CAD build for the part. Positions are in the model's coordinates, mm. A direction names the side the tool comes from. Give positions to 0.01 mm unless a question says otherwise; leave off trailing zeros. Write each loop counter-clockwise with the first axis right and the second up, starting at its lowest first coordinate (ties: lowest second). Pieces come first, ordered by that corner, then holes. Notation, with made-up numbers: M 23,43.5 L 35,43.5 A24 cw 35,76.5 Z; hole C 33,85 d7. An arc over 180 degrees is marked long. One line per question, with ' | ' between items. Start each with the question number.
1. Wall check: L1, parallel to Y at x = 45.5, z = 26.5 (3 decimals); L2, parallel to Z at x = 28, y = 25.5 (3 decimals); L3, parallel to Y at x = 26, z = 20 (3 decimals). Give the ranges that are in metal, low to high.
2. Cut at A-A, the plane z = 22.75. Write the cut outline in (x, y) (3 decimals), then the cut area to 3 significant figures.
3. Pull direction Y, two halves, no side cores. Call faces 1 (the face through (8, 1.905, 16)), 2 (the face through (25, 0, 0)), 3 (the face through (25, 5.08, 20)): released by +Y, released by -Y, zero draft, split by the parting line, or undercut.
4. Flat gauge pins, fed straight in: pin 1 (3.5 mm diameter, centred on x = 30.5, z = 10.5, fed in from -Y) (3 decimals); pin 2 (7 mm diameter, centred on x = 21, z = 13, fed in from -Y) (3 decimals); pin 3 (3.5 mm diameter, centred on x = 41.5, z = 14, fed in from -Y). Where does each tip first touch, or does it go through?
5. Cut at B-B, the plane x = 6.5. Write the cut outline in (y, z) (3 decimals), then the cut area to 3 significant figures.
6. Cut at C-C, the plane y = 26. Write the cut outline in (x, z) (3 decimals), then the cut area to 3 significant figures.
7. Which spindle directions (+Z, -Z, +X, -X, +Y, -Y) get a long thin tool onto all of the face, cutting with end or side? Do faces 4 (the face through (26.612, 1.583, 16.053)), 5 (the face through (25, -22, 3.175)), 6 (the face through (1.293, 1.592, 16.053)). Say none if no direction does.
8. Cut at D-D, the plane z = 8.5. Write the cut outline in (x, y) (3 decimals).
```python
from build123d import *

# Parameters (mm, degrees)
F1_DEPTH = 50.8
F2_SIZE  = 8.89
F4_DEPTH = 25.4


with BuildPart() as f1:
    # F0 (on Right) → F1 (new body)
    with BuildSketch(Plane.YZ):
        Polygon((-30.48, 0), (0, 0), (30.48, 0), (30.48, 3.175), (5.08, 3.175), (5.08, 28.575), (1.905, 28.575), (1.905, 3.175), (0, 3.175), (-1.905, 3.175), (-1.905, 28.575), (-5.08, 28.575), (-5.08, 3.175), (-30.48, 3.175), align=None)
    extrude(amount=F1_DEPTH)

    # F2
    f2_edges = [f1.edges().sort_by_distance(p)[0] for p in [
        (25.4, 5.08, 3.175),
        (25.4, -5.08, 3.175),
    ]]
    chamfer(f2_edges, length=F2_SIZE)

    # F3 (on face) → F4 (join, through all)
    with BuildSketch(Plane.XY.offset(28.575)):
        Polygon((2.54, 1.27), (4.999344, 1.905), (0.080656, 1.905), align=None)
        Polygon((13.97, 1.27), (16.429344, 1.905), (11.510656, 1.905), align=None)
        Polygon((27.859344, 1.905), (25.4, 1.905), (25.4, 1.27), align=None)
        Polygon((25.4, 1.27), (25.4, 1.905), (22.940656, 1.905), align=None)
        Polygon((39.289344, 1.905), (34.370656, 1.905), (36.83, 1.27), align=None)
        Polygon((50.719344, 1.905), (45.800656, 1.905), (48.26, 1.27), align=None)
    extrude(amount=-F4_DEPTH)


solid = f1.part
```
Here are the results:
1) L1: -5.08 to -1.905, 1.905 to 5.08 | L2: 0 to 3.175 | L3: -5.08 to -1.905, 1.425 to 5.08
2) outline: M 0,-5.08 L 50.8,-5.08 L 50.8,-1.905 L 0,-1.905 Z; M 0,1.905 L 0.081,1.905 L 2.54,1.27 L 4.999,1.905 L 11.511,1.905 L 13.97,1.27 L 16.429,1.905 L 22.941,1.905 L 25.4,1.27 L 27.859,1.905 L 34.371,1.905 L 36.83,1.27 L 39.289,1.905 L 45.801,1.905 L 48.26,1.27 L 50.719,1.905 L 50.8,1.905 L 50.8,5.08 L 0,5.08 Z | area: 330 mm^2
3) face 1: undercut | face 2: zero draft | face 3: released by +Y
4) pin 1: y = -8.395 | pin 2: y = -7.645 | pin 3: y = -5.08
5) outline: M -30.48,0 L 30.48,0 L 30.48,3.175 L 13.97,3.175 L 5.08,12.065 L 5.08,28.575 L 1.905,28.575 L 1.905,3.175 L -1.905,3.175 L -1.905,28.575 L -5.08,28.575 L -5.08,12.065 L -13.97,3.175 L -30.48,3.175 Z | area: 434 mm^2
6) outline: M 0,0 L 50.8,0 L 50.8,3.175 L 0,3.175 Z | area: 161 mm^2
7) face 4: +Z | face 5: +Z, +X, -X, -Y | face 6: +Z, -X
8) outline: M 0,-8.645 L 50.8,-8.645 L 50.8,-1.905 L 0,-1.905 Z; M 0,1.905 L 0.081,1.905 L 2.54,1.27 L 4.999,1.905 L 11.511,1.905 L 13.97,1.27 L 16.429,1.905 L 22.941,1.905 L 25.4,1.27 L 27.859,1.905 L 34.371,1.905 L 36.83,1.27 L 39.289,1.905 L 45.801,1.905 L 48.26,1.27 L 50.719,1.905 L 50.8,1.905 L 50.8,8.645 L 0,8.645 Z
